Check sheet for the modelled part. Datum: model origin and axes. Units: mm. A direction names the side the tool comes from. Coordinates: 2 decimals unless noted, no trailing zeros. Loops run counter-clockwise (first coordinate to the right, second up) from the corner with the lowest first, then second, coordinate; pieces in that order, holes last.
Autodesk Inventor part; units mm, degrees
ref_plane "YZ Plane" through (0, 0, 0) normal (1, 0, 0) x (0, 1, 0)
ref_plane "XZ Plane" through (0, 0, 0) normal (0, 1, 0) x (-1, 0, 0)
ref_plane "XY Plane" through (0, 0, 0) normal (0, 0, 1) x (1, 0, 0)
sketch "Sketch1" plane through (0, 0, 0) normal (0, 0, 1) x (1, 0, 0)
  circle A0 centre (0, 0) radius 3.75
  dimension "d0" = 7.5
extrude "Extrusion1" add sketch "Sketch1" against normal blind 5
chamfer "Chamfer1" distance 0.5 angle 45 1 edges at (-3.75, 0, 0) measured on face at (3.7014, -0.6015, -3.3333)
sketch "Sketch2" plane through (0, 0, -5) normal (0, 0, -1) x (-1, 0, 0)
  circle A0 centre (0, 0) radius 2.5
  dimension "d6" = 5
extrude "Extrusion2" add sketch "Sketch2" along normal blind 1
sketch "Sketch3" plane through (0, 0, -6) normal (0, 0, -1) x (-1, 0, 0)
  circle A0 centre (0, 0) radius 3.8
  dimension "d9" = 7.6
extrude "Extrusion3" add sketch "Sketch3" along normal blind 1
sketch "Sketch4" plane through (0, 0, -7) normal (0, 0, -1) x (-1, 0, 0)
  circle A0 centre (0, 0) radius 4
extrude "Extrusion4" add sketch "Sketch4" along normal blind 2
chamfer "Chamfer2" distance 0.5 angle 45 1 edges at (4, 0, -9)
properties part number "Bolt" material "Steel"
1) Section check C-C on z = -4.25. Enter the section's corners in (x, y).
Answer sheet:
outline: circle Ø7.5 at (0, 0)
2) Mould release check, pull along Z, two halves, no side actions. Record for faces 4 (the flat face through (0.9, -2.5, -6)), 5 (the flat face through (0, 0, 0)), 6 (the flat face through (0, 0, -9)): +Z half, -Z half, draft (parallel to the pull), parting line (faces both ways), or undercut.
Answer sheet:
face 4: undercut
face 5: +Z half
face 6: -Z half
3) Scan lines: line 1 (Z direction, x = 2.75, y = 1.25); line 2 (Z direction, x = 2.75, y = 2); line 3 (Y direction, x = -1.25, z = -3.75). Record each from-to range of solid material in increasing order.
Answer sheet:
line 1: z = -9 to -6, -5 to 0
line 2: z = -9 to -6, -5 to -0.15
line 3: y = -3.54 to 3.54
4) Section check A-A on y = 0. Enter the section's corners in (x, z), plus the area to 3 significant figures.
Answer sheet:
outline: (-4, -8.5) - (-3.5, -9) - (3.5, -9) - (4, -8.5) - (4, -7) - (3.8, -7) - (3.8, -6) - (2.5, -6) - (2.5, -5) - (3.75, -5) - (3.75, -0.5) - (3.25, 0) - (-3.25, 0) - (-3.75, -0.5) - (-3.75, -5) - (-2.5, -5) - (-2.5, -6) - (-3.8, -6) - (-3.8, -7) - (-4, -7) - close
area: 65.6 mm2
5) Set-up check for faces 1 (the cylindrical face through (0.867, 3.905, -7.74)), 2 (the flat face through (0, 3, -5)), 3 (the cylindrical face through (-3.746, 0.165, -2.718)): record each of +Z, -Z, +X, -X, +Y, -Y from which the full face is reachable in a straight line by a thin tool's end or side.
Answer sheet:
face 1: +Z, -Z
face 2: none
face 3: +Z
6) Depth check by flat-ended pin: pin 1 (4 mm diameter, centred on y = 2, z = -1, fed in from -X); pin 2 (2 mm diameter, centred on x = 2.5, z = -4, fed in from +Y); pin 3 (1.5 mm diameter, centred on x = 2.5, z = -1.5, fed in from -Y). Enter the tip coordinate at first touch or a pass-through.
Answer sheet:
pin 1: stops at x = -3.75
pin 2: stops at y = 3.44
pin 3: stops at y = -3.32
7) Section check D-D on z = -5.5. Enter the section's corners in (x, y), plus the area to 3 significant figures.
Answer sheet:
outline: circle Ø5 at (0, 0)
area: 19.6 mm2
